Part model, mm, in its own coordinate system. Round coordinates to 2 decimals unless told otherwise and drop trailing zeros. Write each loop counter-clockwise with the first axis right and the second up, starting at its lowest first coordinate (ties: lowest second). Pieces come first, ordered by that corner, then holes. Notation, with made-up numbers: (16, 81) -> (32, 81) arc R26 cw to (32, 108) -> close; hole circle Ø1 at (25.5, 12.25). An arc over 180 degrees is marked (long way). Return JSON: item names as keys, results as strings. Group by question number.
```python
from build123d import *

# Parameters (mm, degrees)
SKETCH1_R           = 2.38125
SKETCH1_R_2         = 9.525
BOSS_EXTRUDE1_DEPTH = 1.5875


with BuildPart() as part:
    # Sketch1 → Boss-Extrude1 (new, symmetric)
    with BuildSketch(Plane(origin=(0, 0, 0), x_dir=(1, 0, 0), z_dir=(0, 1, 0))):
        with BuildLine():
            ThreePointArc((-16.508630953, 23.323716022), (-21.889374295, 21.889374295), (-23.323716022, 16.508630953))
            ThreePointArc((-23.323716022, 16.508630953), (-28.575, 0), (-23.323716022, -16.508630953))
            ThreePointArc((-23.323716022, -16.508630953), (-21.889374295, -21.889374295), (-16.508630953, -23.323716022))
            ThreePointArc((-16.508630953, -23.323716022), (0, -28.575), (16.508630953, -23.323716022))
            ThreePointArc((16.508630953, -23.323716022), (21.889374295, -21.889374295), (23.323716022, -16.508630953))
            ThreePointArc((23.323716022, -16.508630953), (28.575, 0), (23.323716022, 16.508630953))
            ThreePointArc((23.323716022, 16.508630953), (21.889374295, 21.889374295), (16.508630953, 23.323716022))
            ThreePointArc((16.508630953, 23.323716022), (0, 28.575), (-16.508630953, 23.323716022))
        make_face()
        with Locations(Location((-17.960512242, 17.960512242, 0), (0, 0, 270))):
            Circle(SKETCH1_R, mode=Mode.SUBTRACT)
        with Locations(Location((17.960512242, 17.960512242, 0), (0, 0, 90))):
            Circle(SKETCH1_R, mode=Mode.SUBTRACT)
        with Locations(Location((-17.960512242, -17.960512242, 0), (0, 0, 90))):
            Circle(SKETCH1_R, mode=Mode.SUBTRACT)
        with Locations(Location((17.960512242, -17.960512242, 0), (0, 0, 270))):
            Circle(SKETCH1_R, mode=Mode.SUBTRACT)
        with Locations(Location((0, 0, 0), (0, 0, 270))):
            Circle(SKETCH1_R_2, mode=Mode.SUBTRACT)
    extrude(amount=BOSS_EXTRUDE1_DEPTH, both=True)


solid = part.part
```
Item 1: Two-plate mould, pull along X, no slides. Class faces 1 (the face through (-28.574, 0.022, -0.246)), 2 (the face through (-7, 1.588, -7)), 3 (the face through (17.86, -0.02, -15.58)): released by +X, released by -X, zero draft, split by the parting line, or undercut.
Item 2: Cut at C-C (y = -0.65). State how many separate pieces and enclosed holes the cut face has, then the cut area to 3 significant figures.
Item 3: Cut at D-D (x = 14.5). Write the cut outline in (y, z).
Item 4: Cut at A-A (x = 0). Write the cut outline in (y, z) (1 decimal), then the cut area to 3 significant figures.
Item 5: Cut at B-B (z = 0). Write the cut outline in (x, y) (1 decimal).
Item 6: Wall check: L1, parallel to Z at x = -5, y = 0.05; L2, parallel to Z at x = -5.5, y = 1.3; L3, parallel to X at y = -0.15, z = 6. Give the ranges that are in metal, low to high.
Item 7: Flat gauge pins, fed straight in: P1, Ø15, axis at x = 0, z = 0, coming from the -Y side; P2, Ø1.5, axis at x = -6, y = 1, coming from the +Z side. Where does each tip first touch, or does it go through?
Checks:
{
 "1": {"face 1": "released by -X", "face 2": "zero draft", "face 3": "undercut"},
 "2": {"separate pieces": "1", "enclosed holes": "5", "area": "2,270 mm2"},
 "3": {"outline": "(-1.59, -24.62) -> (1.59, -24.62) -> (1.59, 24.62) -> (-1.59, 24.62) -> close"},
 "4": {"outline": "(-1.6, -28.6) -> (1.6, -28.6) -> (1.6, -9.5) -> (-1.6, -9.5) -> close; (-1.6, 9.5) -> (1.6, 9.5) -> (1.6, 28.6) -> (-1.6, 28.6) -> close", "area": "121 mm2"},
 "5": {"outline": "(-28.6, -1.6) -> (-9.5, -1.6) -> (-9.5, 1.6) -> (-28.6, 1.6) -> close; (9.5, -1.6) -> (28.6, -1.6) -> (28.6, 1.6) -> (9.5, 1.6) -> close"},
 "6": {"L1": "z = -28.13 to -8.11, 8.11 to 28.13", "L2": "z = -28.04 to -7.78, 7.78 to 28.04", "L3": "x = -27.94 to -7.4, 7.4 to 27.94"},
 "7": {"P1": "passes through", "P2": "stops at z = 28.09"}
}
